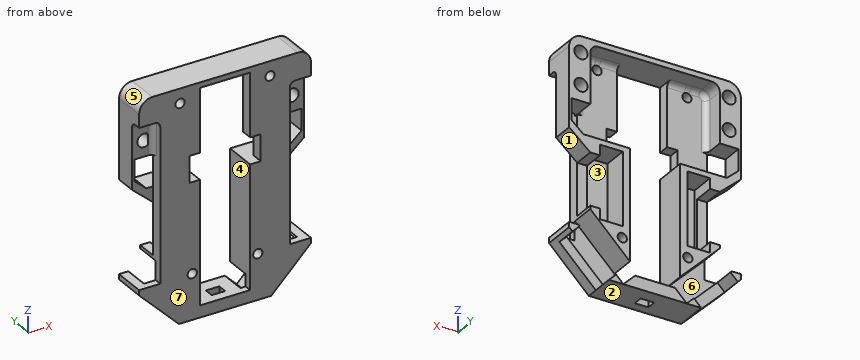
```python
from build123d import *

# Parameters (mm, degrees)
SKETCH1_W               = 70
SKETCH1_H               = 85
BOSS_EXTRUDE1_DEPTH     = 2.8
SKETCH2_W               = 10.5
SKETCH2_H               = 60
CUT_EXTRUDE1_DEPTH      = 10
SKETCH3_W               = 2.519429159
SKETCH3_H               = 8
CUT_EXTRUDE2_DEPTH      = 10
CUT_EXTRUDE3_DEPTH      = 10
BOSS_EXTRUDE2_OUTLINE_W = 8.6
BOSS_EXTRUDE2_OUTLINE_H = 27.6
BOSS_EXTRUDE2_DEPTH     = 1.5
BOSS_EXTRUDE3_DEPTH     = 8
BOSS_EXTRUDE4_DEPTH     = 8
CUT_EXTRUDE5_DEPTH      = 8
SKETCH14_W              = 64.961141682
SKETCH14_H              = 2
BOSS_EXTRUDE5_DEPTH     = 12.3
FILLET1_R               = 5
SKETCH15_W              = 4
SKETCH15_H              = 10
CUT_EXTRUDE8_DEPTH      = 12.7
SKETCH16_R              = 1.75
CUT_EXTRUDE9_DEPTH      = 12.7
FILLET3_R               = 2
FILLET4_R               = 2
FILLET5_R               = 3
FILLET6_R               = 2
SKETCH17_R              = 2.5
CUT_EXTRUDE10_DEPTH     = 8
SKETCH18_W              = 19
SKETCH18_H              = 7
CUT_EXTRUDE11_DEPTH     = 57.451881976
SKETCH19_W              = 5.1
SKETCH19_H              = 3.6
CUT_EXTRUDE12_DEPTH     = 10


# Read off the part's stored shape, not the designer's step: Boss-Extrude2
with BuildPart() as part:
    # Sketch1 → Boss-Extrude1 (new body)
    with BuildSketch(Plane(origin=(0, 0, 0), x_dir=(1, 0, 0), z_dir=(0, 1, 0))):
        Rectangle(SKETCH1_W, SKETCH1_H)
    extrude(amount=BOSS_EXTRUDE1_DEPTH)

    # Sketch2 → Cut-Extrude1 (cut)
    with BuildSketch(Plane(origin=(0, 0, 0), x_dir=(-1, 0, 0), z_dir=(0, -1, 0))):
        with Locations((-29.75, -4.5)):
            Rectangle(SKETCH2_W, SKETCH2_H)
        with Locations((29.75, -4.5)):
            Rectangle(SKETCH2_W, SKETCH2_H)
    extrude(amount=-CUT_EXTRUDE1_DEPTH, mode=Mode.SUBTRACT)

    # Sketch3 → Cut-Extrude2 (cut)
    with BuildSketch(Plane(origin=(0, 2.8, 0), x_dir=(1, 0, 0), z_dir=(0, 1, 0))):
        Polygon((17.462549034, 42.5), (35, 42.5), (35, 25.5), (32.484854108, 25.5), (32.484996169, 27.489999862), align=None)
        with Locations((33.740285421, -38.5)):
            Rectangle(SKETCH3_W, SKETCH3_H)
        with Locations((-33.740285421, -38.5)):
            Rectangle(SKETCH3_W, SKETCH3_H)
        Polygon((-32.484996169, 27.489999862), (-17.462549034, 42.5), (-35, 42.5), (-35, 25.5), (-32.484854108, 25.5), align=None)
    extrude(amount=-CUT_EXTRUDE2_DEPTH, mode=Mode.SUBTRACT)

    # Sketch5 → Cut-Extrude3 (cut)
    with BuildSketch(Plane(origin=(0, 2.8, 0), x_dir=(1, 0, 0), z_dir=(0, 1, 0))):
        Polygon((-9.5, -42.5), (9.5, -42.5), (9.5, 31), (5.25, 31), (5.25, 38), (-5.25, 38), (-5.25, 31), (-9.5, 31), align=None)
    extrude(amount=-CUT_EXTRUDE3_DEPTH, mode=Mode.SUBTRACT)

    # Boss-Extrude2 outline → Boss-Extrude2 (add)
    with BuildSketch(Plane(origin=(0, 2.8, 0), x_dir=(1, 0, 0), z_dir=(0, 1, 0))):
        Polygon((-32.480570841, -42.5), (-9.5, -42.5), (-9.5, 31), (-5.25, 31), (-5.25, 38), (5.25, 38), (5.25, 31), (9.5, 31), (9.5, -42.5), (32.480570841, -42.5), (32.480570841, -34.5), (24.5, -34.5), (24.5, 18.363483562), (6.1866146, 36.661695224), (11.982486603, 42.462373437), (28.958926038, 25.5), (32.484854108, 25.5), (32.484996169, 27.489999862), (17.462549034, 42.5), (-17.462549034, 42.5), (-32.484996169, 27.489999862), (-32.484854108, 25.5), (-28.958926038, 25.5), (-11.982486603, 42.462373437), (-6.1866146, 36.661695224), (-24.5, 18.363483562), (-24.5, -34.5), (-32.480570841, -34.5), align=None)
        with Locations((-16.5, 7.293849796)):
            Rectangle(BOSS_EXTRUDE2_OUTLINE_W, BOSS_EXTRUDE2_OUTLINE_H, mode=Mode.SUBTRACT)
        with Locations((16.5, 7.293849796)):
            Rectangle(BOSS_EXTRUDE2_OUTLINE_W, BOSS_EXTRUDE2_OUTLINE_H, mode=Mode.SUBTRACT)
    extrude(amount=BOSS_EXTRUDE2_DEPTH)

    # Sketch9 → Boss-Extrude3 (add)
    with BuildSketch(Plane(origin=(0, 4.3, 0), x_dir=(1, 0, 0), z_dir=(0, 1, 0))):
        Polygon((-24.5, -34.5), (-32.480570841, -34.5), (-32.480570841, -42.5), (-9.5, -42.5), (-9.5, 31), (-5.25, 31), (-5.25, 38), (0, 38), (5.25, 38), (5.25, 31), (9.5, 31), (9.5, -42.5), (32.480570841, -42.5), (32.480570841, -34.5), (24.5, -34.5), (24.5, -2.556150204), (20.8, -2.556150204), (20.8, -6.506150204), (12.2, -6.506150204), (12.2, 21.093849796), (20.8, 21.093849796), (20.8, 17.143849796), (24.5, 17.143849796), (24.5, 18.363483562), (6.1866146, 36.661695224), (11.982486603, 42.462373437), (14.705975764, 39.74114085), (17.462549034, 42.5), (-17.462549034, 42.5), (-14.705975764, 39.74114085), (-11.982486603, 42.462373437), (-6.1866146, 36.661695224), (-24.5, 18.363483562), (-24.5, 17.143849796), (-20.8, 17.143849796), (-20.8, 21.093849796), (-12.2, 21.093849796), (-12.2, -6.506150204), (-20.8, -6.506150204), (-20.8, -2.556150204), (-24.5, -2.556150204), align=None)
        Polygon((-31.256844783, 28.717133652), (-32.484996169, 27.489999862), (-32.484854108, 25.5), (-28.958926038, 25.5), (-28.500271514, 25.958274502), align=None)
        Polygon((32.484996169, 27.489999862), (31.256844783, 28.717133652), (28.500271514, 25.958274502), (28.958926038, 25.5), (32.484854108, 25.5), align=None)
    extrude(amount=BOSS_EXTRUDE3_DEPTH)

    # Sketch10 → Boss-Extrude4 (add)
    with BuildSketch(Plane(origin=(0, 12.3, 0), x_dir=(1, 0, 0), z_dir=(0, 1, 0))):
        Polygon((-32.480570841, -34.5), (-24.5, -34.5), (-24.5, -2.556150204), (-32.480570841, -9.5), align=None)
        Polygon((32.480570841, -34.5), (24.5, -34.5), (24.5, -9.5), (24.5, -2.556150204), (32.480570841, -9.5), align=None)
    extrude(amount=-BOSS_EXTRUDE4_DEPTH)

    # Sketch11 → Cut-Extrude5 (cut)
    with BuildSketch(Plane(origin=(0, 12.3, 0), x_dir=(1, 0, 0), z_dir=(0, 1, 0))):
        Polygon((-24.480570841, -42.5), (-24.480570841, -20.499611406), (-31.560570841, -20.499611406), (-31.560570841, -12.405434935), (-27.162134436, -8.5), (-9.5, -8.5), (-9.5, -12.405776235), (-9.5, -42.5), align=None)
        Polygon((9.5, -42.5), (24.480570841, -42.5), (24.480570841, -20.499611406), (31.560570841, -20.499611406), (31.560570841, -12.405434935), (27.162134436, -8.5), (9.5, -8.5), (9.5, -12.405776235), align=None)
    extrude(amount=-CUT_EXTRUDE5_DEPTH, mode=Mode.SUBTRACT)

    # Sketch14 → Boss-Extrude5 (add)
    with BuildSketch(Plane(origin=(0, 0, 0), x_dir=(-1, 0, 0), z_dir=(0, -1, 0))):
        with Locations((0, -43.5)):
            Rectangle(SKETCH14_W, SKETCH14_H)
    extrude(amount=-BOSS_EXTRUDE5_DEPTH)

    # Fillet1
    fillet1_edges = [part.edges().sort_by_distance(p)[0] for p in [
        (32.480570841, 6.15, 44.5),
        (-32.480570841, 6.15, 44.5),
    ]]
    fillet(fillet1_edges, radius=FILLET1_R)

    # Sketch15 → Cut-Extrude8 (cut)
    with BuildSketch(Plane(origin=(0, 4.3, 0), x_dir=(1, 0, 0), z_dir=(0, 1, 0))):
        with Locations((-11.5, -13.5)):
            Rectangle(SKETCH15_W, SKETCH15_H)
        with Locations((11.5, -13.5)):
            Rectangle(SKETCH15_W, SKETCH15_H)
    extrude(amount=-CUT_EXTRUDE8_DEPTH, mode=Mode.SUBTRACT)

    # Sketch16 → Cut-Extrude9 (cut)
    with BuildSketch(Plane(origin=(0, 0, 0), x_dir=(-1, 0, 0), z_dir=(0, -1, 0))):
        with Locations(Location((-17.000570841, -39, 0), (0, 0, 90))):
            Circle(SKETCH16_R)
        with Locations(Location((-12.394846918, 25.4, 0), (0, 0, 90))):
            Circle(SKETCH16_R)
        with Locations(Location((12.394846918, 25.4, 0), (0, 0, 270))):
            Circle(SKETCH16_R)
        with Locations(Location((17.000570841, -39, 0), (0, 0, 90))):
            Circle(SKETCH16_R)
    extrude(amount=-CUT_EXTRUDE9_DEPTH, mode=Mode.SUBTRACT)

    # Fillet3
    fillet3_edges = [part.edges().sort_by_distance(p)[0] for p in [
        (-24.5, 4.3, 27.499805703),
        (24.5, 4.3, 27.499805703),
    ]]
    fillet(fillet3_edges, radius=FILLET3_R)

    # Fillet4
    fillet4_edges = [part.edges().sort_by_distance(p)[0] for p in [
        (-29.490285421, 4.3, 34.5),
        (24.5, 1.15, 34.5),
        (29.490285421, 4.3, 34.5),
        (25.085786438, 3.714213562, 34.5),
        (-24.5, 1.15, 34.5),
        (-25.085786438, 3.714213562, 34.5),
    ]]
    fillet(fillet4_edges, radius=FILLET4_R)

    # Fillet5
    fillet5_edges = [part.edges().sort_by_distance(p)[0] for p in [
        (-24.480570841, 8.3, 42.5),
        (24.480570841, 8.3, 42.5),
    ]]
    fillet(fillet5_edges, radius=FILLET5_R)

    # Fillet6
    fillet6_edges = [part.edges().sort_by_distance(p)[0] for p in [
        (-24.480570841, 4.3, 29.999805703),
        (15.490285421, 4.3, 42.5),
        (-15.490285421, 4.3, 42.5),
        (-23.601891185, 4.3, 41.621320344),
        (24.480570841, 4.3, 29.999805703),
        (23.601891185, 4.3, 41.621320344),
    ]]
    fillet(fillet6_edges, radius=FILLET6_R)

    # Sketch17 → Cut-Extrude10 (cut)
    with BuildSketch(Plane(origin=(0, 12.3, 0), x_dir=(1, 0, 0), z_dir=(0, 1, 0))):
        with Locations(Location((-28.020570841, -26.499611406, 0), (0, 0, 270))):
            Circle(SKETCH17_R)
        with Locations(Location((-28.020570841, -38.5, 0), (0, 0, 270))):
            Circle(SKETCH17_R)
        with Locations(Location((28.020570841, -38.5, 0), (0, 0, 90))):
            Circle(SKETCH17_R)
        with Locations(Location((28.020570841, -26.499611406, 0), (0, 0, 232.538489895))):
            Circle(SKETCH17_R)
    extrude(amount=-CUT_EXTRUDE10_DEPTH, mode=Mode.SUBTRACT)

    # Sketch18 → Cut-Extrude11 (cut, through all)
    with BuildSketch(Plane(origin=(0, 12.3, 0), x_dir=(1, 0, 0), z_dir=(0, 1, 0))):
        with Locations((0, 34.5)):
            Rectangle(SKETCH18_W, SKETCH18_H)
    extrude(amount=-CUT_EXTRUDE11_DEPTH, mode=Mode.SUBTRACT)

    # Sketch19 → Cut-Extrude12 (cut)
    with BuildSketch(Plane(origin=(0, 0, -42.5), x_dir=(-1, 0, 0), z_dir=(0, 0, -1))):
        with Locations((0.200058215, 5.5)):
            Rectangle(SKETCH19_W, SKETCH19_H)
    extrude(amount=-CUT_EXTRUDE12_DEPTH, mode=Mode.SUBTRACT)


solid = part.part
```
The listing builds one solid part. Answer for the finished solid, in the listing's coordinates (mm). Face numbers are marked on the shaded views. A direction names the side the tool comes from. Give positions to 0.01 mm unless a question says otherwise; leave off trailing zeros. Order: outer loops, then holes, each group sorted by start corner. A loop starts at its lowest first (then second) coordinate and runs counter-clockwise, first axis right, second up.
Item 1: The part is cut by section D-D, the plane y = 1. Count the separate pieces of the cut face and the enclosed holes in it, and give its area (3 significant figures).
From the geometry:
separate pieces: 1
enclosed holes: 5
area: 2,810 mm2
Item 2: The part is cut by section A-A, the plane x = -6. Give the vertices of the cut face in (y, z), and give its area (4 significant figures).
From the geometry:
outline: (0, -42.5) - (12.3, -42.5) - (12.3, -38) - (0, -38) - close; (0, 42.5) - (12.3, 42.5) - (12.3, 44.5) - (0, 44.5) - close
area: 79.95 mm2
Item 3: Given pin 1 Ø4 at (x, z) = (-28.02, 26.5) entering from +Y; pin 2 Ø1.5 at (y, z) = (2, 1) entering from -X; pin 3 Ø2 at (x, y) = (23, 4) entering from -Z, each flat-ended and moving along its own axis, determine where each tip first touches the part or whether it passes through.
From the geometry:
pin 1: stops at y = 4.3
pin 2: stops at x = -24.5
pin 3: stops at z = -37.97
Item 4: Find the intervals of material crossed by probe 1 along X at (y, z) = (9.5, 38.5); probe 2 along X at (y, z) = (3.75, 37.5); probe 3 along X at (y, z) = (7.5, 22), in increasing order.
From the geometry:
probe 1: x = -32.48 to -30.52, -25.52 to -24.48, 24.48 to 25.52, 30.52 to 32.48
probe 2: x = -32.48 to -17.9, -16.1 to -9.5, 9.5 to 16.1, 17.9 to 32.48
probe 3: x = -32.48 to -24.48, 24.48 to 32.48
Item 5: Which of the six approach directions +Z, -Z, +X, -X, +Y, -Y give full straight-line access (tool end or side, diameter ignored) to the marked faces 1, 2, 3 and 4?
From the geometry:
face 1: +X, +Y, -Y
face 2: -Z, +X, -X, +Y, -Y
face 3: +Y
face 4: +Y, -Y
Item 6: For a pull along X with two mould halves and no side action, classify the marked faces 5, 6 and 7 as pulls with the +X half, pulls with the -X half, needs draft (parallel to the pull), parting line crosses it, or undercut.
From the geometry:
face 5: pulls with the -X half
face 6: undercut
face 7: needs draft
Item 7: The part is cut by section C-C, the plane z = -22.5. Give the vertices of the cut face in (x, y), and give its area (3 significant figures).
From the geometry:
outline: (-24.5, 0) - (-9.5, 0) - (-9.5, 12.3) - (-20.36, 12.3) - (-20.36, 2.8) - (-24.5, 2.8) - close; (9.5, 0) - (24.5, 0) - (24.5, 2.8) - (20.36, 2.8) - (20.36, 12.3) - (9.5, 12.3) - close
area: 290 mm2
Item 8: The part is cut by section B-B, the plane z = 16. Give the vertices of the cut face in (x, y).
From the geometry:
outline: (-32.48, 4.3) - (-31.56, 4.3) - (-31.56, 12.3) - (-32.48, 12.3) - close; (-24.5, 0) - (-13.5, 0) - (-13.5, 4.3) - (-24.5, 4.3) - close; (13.5, 0) - (24.5, 0) - (24.5, 4.3) - (13.5, 4.3) - close; (31.56, 4.3) - (32.48, 4.3) - (32.48, 12.3) - (31.56, 12.3) - close
